Input: part model. Units: mm. Frame: model coordinates. A direction names the side the tool comes from. Give positions to 0.01 mm unless a question says otherwise; leave off trailing zeros. Loops run counter-clockwise (first coordinate to the right, second up) from the corner with the lowest first, then second, coordinate; pieces in that order, holes last. Notation, with made-up numbers: (-10, -18.75) - (43, -18.75) arc R14 cw to (43, -12.75) - close; hole circle Ø4 at (47, -38.75). An arc over 180 degrees is marked (long way). One line per question, with ' | ' between items. Start each with the question number.
from build123d import *

# Parameters (mm, degrees)
SZKIC1_R                    = 1.65
SZKIC1_R_2                  = 1.5
SZKIC1_R_3                  = 8.3
DODANIE_WYCI_GNI_CIE1_DEPTH = 6
SFAZOWANIE1_SIZE            = 2
SZKIC2_R                    = 1.65
SZKIC2_R_2                  = 1.5
DODANIE_WYCI_GNI_CIE2_DEPTH = 0.2


with BuildPart() as part:
    # Szkic1 → Dodanie-wyciągnięcie1 (new body)
    with BuildSketch(Plane(origin=(0, 0, 0), x_dir=(1, 0, 0), z_dir=(0, 1, 0))):
        with BuildLine():
            Line((-25.903523773, -8.493281025), (-19.491546416, -8.493281025))
            ThreePointArc((-19.491546416, -8.493281025), (-14.649908292, -7.690412435), (-10.326563391, -5.367753061))
            Line((-10.326563391, -5.367753061), (-8.006357575, -3.576966334))
            ThreePointArc((-8.006357575, -3.576966334), (-7.813323472, -3.431665275), (-7.616835373, -3.29107015))
            ThreePointArc((-7.616835373, -3.29107015), (-2.898841628, 2.073604214), (-1.197535095, 9.012246163))
            Line((-1.197535095, 9.012246163), (-1.197535095, 31.001191788))
            ThreePointArc((-1.197535095, 31.001191788), (-2.898841628, 37.939833736), (-7.616835373, 43.3045081))
            ThreePointArc((-7.616835373, 43.3045081), (-7.813323472, 43.445103226), (-8.006357575, 43.590404284))
            Line((-8.006357575, 43.590404284), (-10.326563391, 45.381191012))
            ThreePointArc((-10.326563391, 45.381191012), (-14.649908292, 47.703850385), (-19.491546416, 48.506718975))
            Line((-19.491546416, 48.506718975), (-25.903523773, 48.506718975))
            ThreePointArc((-25.903523773, 48.506718975), (-30.745161897, 47.703850385), (-35.068506799, 45.381191012))
            Line((-35.068506799, 45.381191012), (-37.388712614, 43.590404284))
            ThreePointArc((-37.388712614, 43.590404284), (-37.581746717, 43.445103226), (-37.778234817, 43.3045081))
            ThreePointArc((-37.778234817, 43.3045081), (-42.496228561, 37.939833736), (-44.197535095, 31.001191788))
            Line((-44.197535095, 31.001191788), (-44.197535095, 9.012246163))
            ThreePointArc((-44.197535095, 9.012246163), (-42.496228561, 2.073604214), (-37.778234817, -3.29107015))
            ThreePointArc((-37.778234817, -3.29107015), (-37.581746717, -3.431665275), (-37.388712614, -3.576966334))
            Line((-37.388712614, -3.576966334), (-35.068506799, -5.367753061))
            ThreePointArc((-35.068506799, -5.367753061), (-30.745161897, -7.690412435), (-25.903523773, -8.493281025))
        make_face()
        with Locations(Location((-38.197535095, 35.506718975, 0), (0, 0, 270))):
            Circle(SZKIC1_R, mode=Mode.SUBTRACT)
        with Locations(Location((-26.047535095, 45.006718975, 0), (0, 0, 270))):
            Circle(SZKIC1_R_2, mode=Mode.SUBTRACT)
        with Locations(Location((-7.197535095, 35.506718975, 0), (0, 0, 270))):
            Circle(SZKIC1_R, mode=Mode.SUBTRACT)
        with Locations(Location((-38.197535095, 4.506718975, 0), (0, 0, 270))):
            Circle(SZKIC1_R, mode=Mode.SUBTRACT)
        with Locations(Location((-26.047535095, -4.993281025, 0), (0, 0, 270))):
            Circle(SZKIC1_R_2, mode=Mode.SUBTRACT)
        with Locations(Location((-7.197535095, 4.506718975, 0), (0, 0, 270))):
            Circle(SZKIC1_R, mode=Mode.SUBTRACT)
        with Locations(Location((-22.697535095, 20.006718975, 0), (0, 0, 270))):
            Circle(SZKIC1_R_3, mode=Mode.SUBTRACT)
    extrude(amount=DODANIE_WYCI_GNI_CIE1_DEPTH)

    # Sfazowanie1
    # the kernel refuses this chamfer: 2 mm, written as the material it takes off along each edge
    with BuildSketch(Plane(origin=(-19.491546416, 6, -33.506718975), x_dir=(0.6109988683682814, 0, -0.791631469089424), z_dir=(0.791631469089424, 0, 0.6109988683682814))) as sfazowanie1_piece_1:
        Polygon((15, -SFAZOWANIE1_SIZE), (15 - SFAZOWANIE1_SIZE, 0), (15, 0), align=None)
    revolve(axis=Axis((-19.491546416, 6, -33.506718975), (0, 1, 0)), revolution_arc=37.661762745, mode=Mode.SUBTRACT)
    with BuildSketch(Plane(origin=(-19.491546416, 6, -48.506718975), x_dir=(0, -0.9996219169112968, -0.02749587661058563), z_dir=(-1, 0, 0)), Plane(origin=(-25.903523773, 6, 8.493281025), x_dir=(0, -0.9996219169112968, 0.027495876610586487), z_dir=(1, 0, 0))) as sfazowanie1_piece_2:
        Polygon((SFAZOWANIE1_SIZE * 0.999621916911, SFAZOWANIE1_SIZE * 0.0274958766106), (-SFAZOWANIE1_SIZE * 0.0274958766106, SFAZOWANIE1_SIZE * 0.999621916911), (0, 0), align=None)
    extrude(amount=6.411977357, mode=Mode.SUBTRACT)
    with BuildSketch(Plane(origin=(-25.903523773, 6, -33.506718975), x_dir=(0, 0, -1), z_dir=(1, 0, 0))) as sfazowanie1_piece_3:
        Polygon((15, -SFAZOWANIE1_SIZE), (15 - SFAZOWANIE1_SIZE, 0), (15, 0), align=None)
    revolve(axis=Axis((-25.903523773, 6, -33.506718975), (0, 1, 0)), revolution_arc=37.661762745, mode=Mode.SUBTRACT)
    with BuildSketch(Plane(origin=(-35.068506799, 6, -45.381191012), x_dir=(-0.01679994949386156, -0.9996219169112968, -0.021766601195139172), z_dir=(-0.7916314690894233, 0, 0.6109988683682824)), Plane(origin=(-37.388712614, 6, 3.576966334), x_dir=(-0.01679994949386157, -0.9996219169112968, 0.02176660119513917), z_dir=(0.791631469089423, 0, 0.6109988683682828)), Plane(origin=(-10.326563391, 6, 5.367753061), x_dir=(0.016799949493862203, -0.9996219169112968, 0.021766601195140015), z_dir=(0.7916314690894233, 0, -0.6109988683682822)), Plane(origin=(-8.006357575, 6, -43.590404284), x_dir=(0.01679994949386218, -0.9996219169112968, -0.02176660119514003), z_dir=(-0.791631469089424, 0, -0.6109988683682814))) as sfazowanie1_piece_4:
        Polygon((SFAZOWANIE1_SIZE * 0.999621916911, SFAZOWANIE1_SIZE * 0.0274958766106), (-SFAZOWANIE1_SIZE * 0.0274958766106, SFAZOWANIE1_SIZE * 0.999621916911), (0, 0), align=None)
    extrude(amount=2.930916602, mode=Mode.SUBTRACT)
    with BuildSketch(Plane(origin=(-43.498701298, 6, -51.506718975), x_dir=(0.6109988683682784, 0, 0.7916314690894262), z_dir=(0.7916314690894262, 0, -0.6109988683682784))) as sfazowanie1_piece_5:
        Polygon((10, SFAZOWANIE1_SIZE), (10 + SFAZOWANIE1_SIZE, 0), (10, 0), align=None)
    revolve(axis=Axis((-43.498701298, 6, -51.506718975), (0, -1, 0)), revolution_arc=2.76869433, mode=Mode.SUBTRACT)
    with BuildSketch(Plane(origin=(-29.197535095, 6, -31.001191788), x_dir=(-0.5720466481227963, 0, -0.820221087494996), z_dir=(0.820221087494996, 0, -0.5720466481227963))) as sfazowanie1_piece_6:
        Polygon((15, -SFAZOWANIE1_SIZE), (15 - SFAZOWANIE1_SIZE, 0), (15, 0), align=None)
    revolve(axis=Axis((-29.197535095, 6, -31.001191788), (0, 1, 0)), revolution_arc=55.106931585, mode=Mode.SUBTRACT)
    with BuildSketch(Plane(origin=(-44.197535095, 6, -31.001191788), x_dir=(-0.02749587661058563, -0.9996219169112968, 0), z_dir=(0, 0, 1)), Plane(origin=(-1.197535095, 6, -9.012246163), x_dir=(0.027495876610586382, -0.9996219169112968, 0), z_dir=(0, 0, -1))) as sfazowanie1_piece_7:
        Polygon((SFAZOWANIE1_SIZE * 0.999621916911, SFAZOWANIE1_SIZE * 0.0274958766106), (-SFAZOWANIE1_SIZE * 0.0274958766106, SFAZOWANIE1_SIZE * 0.999621916911), (0, 0), align=None)
    extrude(amount=21.988945625, mode=Mode.SUBTRACT)
    with BuildSketch(Plane(origin=(-29.197535095, 6, -9.012246163), x_dir=(-1, 0, 0), z_dir=(0, 0, -1))) as sfazowanie1_piece_8:
        Polygon((15, -SFAZOWANIE1_SIZE), (15 - SFAZOWANIE1_SIZE, 0), (15, 0), align=None)
    revolve(axis=Axis((-29.197535095, 6, -9.012246163), (0, 1, 0)), revolution_arc=55.106931585, mode=Mode.SUBTRACT)
    with BuildSketch(Plane(origin=(-43.498701298, 6, 11.493281025), x_dir=(0.5720466481228126, 0, -0.8202210874949846), z_dir=(-0.8202210874949846, 0, -0.5720466481228126))) as sfazowanie1_piece_9:
        Polygon((10, SFAZOWANIE1_SIZE), (10 + SFAZOWANIE1_SIZE, 0), (10, 0), align=None)
    revolve(axis=Axis((-43.498701298, 6, 11.493281025), (0, -1, 0)), revolution_arc=2.76869433, mode=Mode.SUBTRACT)
    with BuildSketch(Plane(origin=(-25.903523773, 6, -6.506718975), x_dir=(-0.6109988683682754, 0, 0.7916314690894285), z_dir=(-0.7916314690894285, 0, -0.6109988683682754))) as sfazowanie1_piece_10:
        Polygon((15, -SFAZOWANIE1_SIZE), (15 - SFAZOWANIE1_SIZE, 0), (15, 0), align=None)
    revolve(axis=Axis((-25.903523773, 6, -6.506718975), (0, 1, 0)), revolution_arc=37.661762745, mode=Mode.SUBTRACT)
    with BuildSketch(Plane(origin=(-19.491546416, 6, -6.506718975), x_dir=(0, 0, 1), z_dir=(-1, 0, 0))) as sfazowanie1_piece_11:
        Polygon((15, -SFAZOWANIE1_SIZE), (15 - SFAZOWANIE1_SIZE, 0), (15, 0), align=None)
    revolve(axis=Axis((-19.491546416, 6, -6.506718975), (0, 1, 0)), revolution_arc=37.661762745, mode=Mode.SUBTRACT)
    with BuildSketch(Plane(origin=(-1.896368892, 6, 11.493281025), x_dir=(-0.61099886836827, 0, -0.7916314690894327), z_dir=(-0.7916314690894327, 0, 0.61099886836827))) as sfazowanie1_piece_12:
        Polygon((10, SFAZOWANIE1_SIZE), (10 + SFAZOWANIE1_SIZE, 0), (10, 0), align=None)
    revolve(axis=Axis((-1.896368892, 6, 11.493281025), (0, -1, 0)), revolution_arc=2.76869433, mode=Mode.SUBTRACT)
    with BuildSketch(Plane(origin=(-16.197535095, 6, -9.012246163), x_dir=(0.5720466481227972, 0, 0.8202210874949952), z_dir=(-0.8202210874949952, 0, 0.5720466481227972))) as sfazowanie1_piece_13:
        Polygon((15, -SFAZOWANIE1_SIZE), (15 - SFAZOWANIE1_SIZE, 0), (15, 0), align=None)
    revolve(axis=Axis((-16.197535095, 6, -9.012246163), (0, 1, 0)), revolution_arc=55.106931585, mode=Mode.SUBTRACT)
    with BuildSketch(Plane(origin=(-16.197535095, 6, -31.001191788), x_dir=(1, 0, 0), z_dir=(0, 0, 1))) as sfazowanie1_piece_14:
        Polygon((15, -SFAZOWANIE1_SIZE), (15 - SFAZOWANIE1_SIZE, 0), (15, 0), align=None)
    revolve(axis=Axis((-16.197535095, 6, -31.001191788), (0, 1, 0)), revolution_arc=55.106931585, mode=Mode.SUBTRACT)
    with BuildSketch(Plane(origin=(-1.896368892, 6, -51.506718975), x_dir=(-0.5720466481227885, 0, 0.8202210874950013), z_dir=(0.8202210874950013, 0, 0.5720466481227885))) as sfazowanie1_piece_15:
        Polygon((10, SFAZOWANIE1_SIZE), (10 + SFAZOWANIE1_SIZE, 0), (10, 0), align=None)
    revolve(axis=Axis((-1.896368892, 6, -51.506718975), (0, -1, 0)), revolution_arc=2.76869433, mode=Mode.SUBTRACT)

    # Szkic2 → Dodanie-wyciągnięcie2 (add)
    with BuildSketch(Plane.XZ):
        with Locations(Location((-38.197535095, -35.506718975, 0), (0, 0, 270))):
            Circle(SZKIC2_R)
        with Locations(Location((-26.047535095, -45.006718975, 0), (0, 0, 270))):
            Circle(SZKIC2_R_2)
        with Locations(Location((-7.197535095, -35.506718975, 0), (0, 0, 270))):
            Circle(SZKIC2_R)
        with Locations(Location((-7.197535095, -4.506718975, 0), (0, 0, 270))):
            Circle(SZKIC2_R)
        with Locations(Location((-38.197535095, -4.506718975, 0), (0, 0, 270))):
            Circle(SZKIC2_R)
        with Locations(Location((-26.047535095, 4.993281025, 0), (0, 0, 270))):
            Circle(SZKIC2_R_2)
    extrude(amount=-DODANIE_WYCI_GNI_CIE2_DEPTH)


solid = part.part
Q1. Section A-A, the plane y = 1. Output: boundary loops of the cut face in (x, z), plus the area to 3 significant figures.
Q2. Section B-B, the plane z = -13. Output: boundary loops of the cut face in (x, y), plus the area to 3 significant figures.
Q3. Draft query along Z for faces 1 (the face through (-22.742, 4.986, 7.507)), 2 (the face through (-14.99, 5.24, -46.51)), 3 (the face through (-7, 0.2, -4)). Return one class per face: +Z half, -Z half, draft (parallel to the pull), parting line (faces both ways), or undercut.
Q4. Section D-D, the plane z = -24. Output: boundary loops of the cut face in (x, y).
Q5. First-contact query: pin 1 (1.6 mm diameter, centred on x = -8, z = -35, fed in from +Y); pin 2 (2.5 mm diameter, centred on x = -38.2, z = -35.51, fed in from +Y). Flat tips, straight axial feed; report the tip coordinate or a pass-through.
Q6. Line query: L1, parallel to Z at x = -22.5, y = 2; L2, parallel to Z at x = -26, y = 2.75; L3, parallel to X at y = 2.5, z = -36. Output: solid intervals per line, ascending. Write a range as from..to.
Q7. Section C-C, the plane y = 4.75. Output: boundary loops of the cut face in (x, z).
Q8. Access query for faces 4 (the face through (-44.198, 2, -20)), 5 (the face through (-7, 0.2, -35)). Directions: +Z, -Z, +X, -X, +Y, -Y. A direction counts if a zero-diameter tool reaches every point of the face in a straight line with its end or side. Return the directions, or none.
Solved:
1) outline: (-44.2, -31) arc R15 ccw to (-37.78, -43.3) arc R10 cw to (-37.39, -43.59) - (-35.07, -45.38) arc R15 ccw to (-25.9, -48.51) - (-19.49, -48.51) arc R15 ccw to (-10.33, -45.38) - (-8.01, -43.59) arc R10 cw to (-7.62, -43.3) arc R15 ccw to (-1.2, -31) - (-1.2, -9.01) arc R15 ccw to (-7.62, 3.29) arc R10 cw to (-8.01, 3.58) - (-10.33, 5.37) arc R15 ccw to (-19.49, 8.49) - (-25.9, 8.49) arc R15 ccw to (-35.07, 5.37) - (-37.39, 3.58) arc R10 cw to (-37.78, 3.29) arc R15 ccw to (-44.2, -9.01) - close; hole circle Ø3.3 at (-38.2, -35.51); hole circle Ø3.3 at (-38.2, -4.51); hole circle Ø16.6 at (-22.7, -20.01); hole circle Ø3 at (-26.05, -45.01); hole circle Ø3 at (-26.05, 4.99); hole circle Ø3.3 at (-7.2, -35.51); hole circle Ø3.3 at (-7.2, -4.51) | area: 1,880 mm²
2) outline: (-44.2, 0) - (-27.15, 0) - (-27.15, 6) - (-42.2, 6) - (-44.2, 4) - close; (-18.25, 0) - (-1.2, 0) - (-1.2, 4) - (-3.2, 6) - (-18.25, 6) - close | area: 201 mm²
3) face 1: +Z half | face 2: -Z half | face 3: undercut
4) outline: (-44.2, 0) - (-29.97, 0) - (-29.97, 6) - (-42.2, 6) - (-44.2, 4) - close; (-15.42, 0) - (-1.2, 0) - (-1.2, 4) - (-3.2, 6) - (-15.42, 6) - close
5) pin 1: stops at y = 6 | pin 2: stops at y = 0.2
6) L1: z = -48.51..-28.3, -11.71..8.49 | L2: z = -48.51..-46.51, -43.51..-27.62, -12.39..3.49, 6.49..8.49 | L3: x = -43.34..-39.77, -36.62..-8.77, -5.62..-2.05
7) outline: (-43.45, -31) arc R14.25 ccw to (-37.35, -42.69) arc R10.75 cw to (-36.93, -43) - (-34.61, -44.79) arc R14.25 ccw to (-25.9, -47.76) - (-19.49, -47.76) arc R14.25 ccw to (-10.78, -44.79) - (-8.46, -43) arc R10.75 cw to (-8.05, -42.69) arc R14.25 ccw to (-1.95, -31) - (-1.95, -9.01) arc R14.25 ccw to (-8.05, 2.68) arc R10.75 cw to (-8.46, 2.98) - (-10.78, 4.77) arc R14.25 ccw to (-19.49, 7.74) - (-25.9, 7.74) arc R14.25 ccw to (-34.61, 4.77) - (-36.93, 2.98) arc R10.75 cw to (-37.35, 2.68) arc R14.25 ccw to (-43.45, -9.01) - close; hole circle Ø3.3 at (-38.2, -35.51); hole circle Ø3.3 at (-38.2, -4.51); hole circle Ø16.6 at (-22.7, -20.01); hole circle Ø3 at (-26.05, -45.01); hole circle Ø3 at (-26.05, 4.99); hole circle Ø3.3 at (-7.2, -35.51); hole circle Ø3.3 at (-7.2, -4.51)
8) face 4: +Z, -Z, -X, +Y, -Y | face 5: +Y
